Geometry: final body of the model. Coordinates: model frame, mm. Give positions to 0.01 mm unless a question says otherwise; leave off trailing zeros. Write each loop counter-clockwise with the first axis right and the second up, starting at its lowest first coordinate (ties: lowest second). Pieces come first, ordered by that corner, then holes. Notation, with made-up numbers: (12.25, -9) -> (67.25, -9) arc R12 ccw to (67.25, 8) -> close; hole circle Ø4 at (55, 75.5). An arc over 180 degrees is marked (long way). Answer as a JSON object with one key per item and string values. Group by question number.
(1) Section query D-D on x = -99.5. Output: boundary loops of the cut face in (y, z), plus the area to 3 significant figures.
(2) Section query C-C on y = 2.05. State how many separate pieces and enclosed holes the cut face has, plus the area to 3 significant figures.
(3) Section query A-A on x = 1.5. Output: boundary loops of the cut face in (y, z), plus the area to 3 significant figures.
(4) Section query B-B on z = -8.5. Output: boundary loops of the cut face in (x, y).
(5) Material intervals for probe 1 along X at (y, z) = (0.65, -19.5); probe 2 along X at (y, z) = (2.1, 30); probe 3 along Z at (x, y) = (-160, 1), sorted ascending.
from build123d import *

# Parameters (mm, degrees)
SKETCH1_R               = 1.6
SKETCH1_W               = 167
SKETCH1_H               = 65
BOSS_EXTRUDE1_DEPTH     = 3
CUT_EXTRUDE1_DEPTH      = 197.104283482
CUT_EXTRUDE1_DEPTH_BACK = 197.104283482
SKETCH2_R               = 1.9
SKETCH2_W               = 13.670656581
SKETCH2_H               = 96.241422334
SKETCH3_R               = 1.9
CUT_EXTRUDE4_DEPTH      = 10
SKETCH7_R               = 1.5
CUT_EXTRUDE5_DEPTH      = 10
STAND_MOUNT_HOLES_DEPTH = 197.104283482


with BuildPart() as part:
    # Sketch1 → Boss-Extrude1 (new body)
    with BuildSketch(Plane(origin=(0, 0, 0), x_dir=(1, 0, 0), z_dir=(0, 1, 0))):
        Polygon((181.5, -30), (165, -50), (70, -50), (70, -74.2), (-70, -74.2), (-70, -50), (-165, -50), (-181.5, -30), (-181.5, 30), (-165, 50), (-70, 50), (-70, 74.2), (70, 74.2), (70, 50), (165, 50), (181.5, 30), align=None)
        with Locations(Location((-35, -58, 0), (0, 0, 270))):
            Circle(SKETCH1_R, mode=Mode.SUBTRACT)
        with Locations(Location((-35, 58, 0), (0, 0, 270))):
            Circle(SKETCH1_R, mode=Mode.SUBTRACT)
        with Locations(Location((35, 58, 0), (0, 0, 270))):
            Circle(SKETCH1_R, mode=Mode.SUBTRACT)
        with Locations(Location((35, -58, 0), (0, 0, 270))):
            Circle(SKETCH1_R, mode=Mode.SUBTRACT)
        with Locations(Location((-80, 38.5, 0), (0, 0, 270))):
            Circle(SKETCH1_R, mode=Mode.SUBTRACT)
        with Locations(Location((-80, -38.5, 0), (0, 0, 270))):
            Circle(SKETCH1_R, mode=Mode.SUBTRACT)
        with Locations(Location((-47.5, 46.5, 0), (0, 0, 270))):
            Circle(SKETCH1_R, mode=Mode.SUBTRACT)
        with Locations(Location((52.5, 46.5, 0), (0, 0, 270))):
            Circle(SKETCH1_R, mode=Mode.SUBTRACT)
        with Locations(Location((52.5, -46.5, 0), (0, 0, 270))):
            Circle(SKETCH1_R, mode=Mode.SUBTRACT)
        with Locations(Location((-47.5, -46.5, 0), (0, 0, 270))):
            Circle(SKETCH1_R, mode=Mode.SUBTRACT)
        with Locations((-7, 0)):
            Rectangle(SKETCH1_W, SKETCH1_H, mode=Mode.SUBTRACT)
    extrude(amount=BOSS_EXTRUDE1_DEPTH)

    # Sketch2 → Cut-Extrude1 (cut, two sides: drawn at the far end of the back side and taken through both)
    with BuildSketch(Plane(origin=(0, 3, 0), x_dir=(1, 0, 0), z_dir=(0, 1, 0)).offset(-CUT_EXTRUDE1_DEPTH_BACK)):
        with Locations(Location((167.5, -30, 0), (0, 0, 270))):
            Circle(SKETCH2_R)
        with Locations(Location((167.5, 30, 0), (0, 0, 270))):
            Circle(SKETCH2_R)
        with Locations(Location((-173.5, 20, 0), (0, 0, 270))):
            Circle(SKETCH2_R)
        with Locations(Location((-173.5, -20, 0), (0, 0, 270))):
            Circle(SKETCH2_R)
        with Locations((182.335328291, -4.374610106)):
            Rectangle(SKETCH2_W, SKETCH2_H)
    extrude(amount=CUT_EXTRUDE1_DEPTH + CUT_EXTRUDE1_DEPTH_BACK, mode=Mode.SUBTRACT)

    # Sketch3 → Cut-Extrude4 (cut)
    with BuildSketch(Plane(origin=(0, 3, 0), x_dir=(1, 0, 0), z_dir=(0, 1, 0))):
        with Locations(Location((-164.5, 24.5, 0), (0, 0, 270))):
            Circle(SKETCH3_R)
        with Locations(Location((-106.5, 24.5, 0), (0, 0, 270))):
            Circle(SKETCH3_R)
        with Locations(Location((-106.5, -24.5, 0), (0, 0, 270))):
            Circle(SKETCH3_R)
        with Locations(Location((-164.5, -24.5, 0), (0, 0, 270))):
            Circle(SKETCH3_R)
        with Locations(Location((-160, 43.75, 0), (0, 0, 270))):
            Circle(SKETCH3_R)
        with Locations(Location((-160, -43.75, 0), (0, 0, 270))):
            Circle(SKETCH3_R)
    extrude(amount=-CUT_EXTRUDE4_DEPTH, mode=Mode.SUBTRACT)

    # Sketch7 → Cut-Extrude5 (cut)
    with BuildSketch(Plane(origin=(0, 3, 0), x_dir=(1, 0, 0), z_dir=(0, 1, 0))):
        with Locations(Location((104.5, 19.5, 0), (0, 0, 270))):
            Circle(SKETCH7_R)
        with Locations(Location((158.5, 30, 0), (0, 0, 270))):
            Circle(SKETCH7_R)
        with Locations(Location((158.5, -30, 0), (0, 0, 270))):
            Circle(SKETCH7_R)
        with Locations(Location((104.5, -19.5, 0), (0, 0, 270))):
            Circle(SKETCH7_R)
    extrude(amount=-CUT_EXTRUDE5_DEPTH, mode=Mode.SUBTRACT)

    # Sketch8 → Stand mount holes (cut, through all)
    with BuildSketch(Plane(origin=(0, 3, 0), x_dir=(1, 0, 0), z_dir=(0, 1, 0))):
        with BuildLine():
            Line((-56, -63.95), (-33.5, -63.95))
            ThreePointArc((-33.5, -63.95), (-30.25, -67.2), (-33.5, -70.45))
            Line((-33.5, -70.45), (-56, -70.45))
            ThreePointArc((-56, -70.45), (-59.25, -67.2), (-56, -63.95))
        make_face()
        with BuildLine():
            Line((33.5, -63.95), (56, -63.95))
            ThreePointArc((56, -63.95), (59.25, -67.2), (56, -70.45))
            Line((56, -70.45), (33.5, -70.45))
            ThreePointArc((33.5, -70.45), (30.25, -67.2), (33.5, -63.95))
        make_face()
        with BuildLine():
            Line((-56, 69.45), (-33.5, 69.45))
            ThreePointArc((-33.5, 69.45), (-30.25, 66.2), (-33.5, 62.95))
            Line((-33.5, 62.95), (-56, 62.95))
            ThreePointArc((-56, 62.95), (-59.25, 66.2), (-56, 69.45))
        make_face()
        with BuildLine():
            Line((33.5, 69.45), (56, 69.45))
            ThreePointArc((56, 69.45), (59.25, 66.2), (56, 62.95))
            Line((56, 62.95), (33.5, 62.95))
            ThreePointArc((33.5, 62.95), (30.25, 66.2), (33.5, 69.45))
        make_face()
    extrude(amount=-STAND_MOUNT_HOLES_DEPTH, mode=Mode.SUBTRACT)


solid = part.part
Answer list:
{
 "1": {"outline": "(0, -50) -> (3, -50) -> (3, 50) -> (0, 50) -> close", "area": "300 mm2"},
 "2": {"separate pieces": "1", "enclosed holes": "29", "area": "30,200 mm2"},
 "3": {"outline": "(0, -74.2) -> (3, -74.2) -> (3, -32.5) -> (0, -32.5) -> close; (0, 32.5) -> (3, 32.5) -> (3, 74.2) -> (0, 74.2) -> close", "area": "250 mm2"},
 "4": {"outline": "(-181.5, 0) -> (-90.5, 0) -> (-90.5, 3) -> (-181.5, 3) -> close; (76.5, 0) -> (175.5, 0) -> (175.5, 3) -> (76.5, 3) -> close"},
 "5": {"probe 1": "-181.5 to -175.33, -171.67 to -90.5, 76.5 to 103, 106 to 175.5", "probe 2": "-181.5 to -90.5, 76.5 to 157, 160 to 165.6, 169.4 to 175.5", "probe 3": "-50 to -45.65, -41.85 to 41.85, 45.65 to 50"}
}
